Design review of the part built by this model. Coordinates are the model's own, in mm. Face numbers are marked on the shaded views. A direction names the side the tool comes from. Give positions to 0.01 mm unless a question says otherwise; leave off trailing zeros. Return JSON: item names as keys, results as strings.
```python
from build123d import *

# Parameters (mm, degrees)
F0_R      = 14.5
F1_DEPTH  = 10
F2_R      = 11.5
F3_DEPTH  = 9
F4_R      = 14.5
F4_R_2    = 11.5
F5_DEPTH  = 6
F6_R      = 25
F7_DEPTH  = 9
F8_R      = 1
F9_R      = 5.75
F10_DEPTH = 12.5
F11_R     = 3.75
F12_DEPTH = 8
F13_SIZE  = 0.5
F14_R     = 2.75
F15_DEPTH = 19


with BuildPart() as f1:
    # F0 (on Top) → F1 (new body)
    with BuildSketch(Plane.XY):
        Circle(F0_R)
    extrude(amount=F1_DEPTH)

    # F2 (on face) → F3 (join)
    with BuildSketch(Plane.XY.offset(10)):
        Circle(F2_R)
        with BuildLine():
            ThreePointArc((2, 7.7459666924), (5.6568542495, 5.6568542495), (7.7459666924, 2))
            Line((7.7459666924, 2), (8.3459666924, 2))
            ThreePointArc((8.3459666924, 2), (10.3459666924, 0), (8.3459666924, -2))
            Line((8.3459666924, -2), (7.7459666924, -2))
            ThreePointArc((7.7459666924, -2), (5.6568542495, -5.6568542495), (2, -7.7459666924))
            Line((2, -7.7459666924), (2, -8.3459666924))
            ThreePointArc((2, -8.3459666924), (0, -10.3459666924), (-2, -8.3459666924))
            Line((-2, -8.3459666924), (-2, -7.7459666924))
            ThreePointArc((-2, -7.7459666924), (-5.6568542495, -5.6568542495), (-7.7459666924, -2))
            Line((-7.7459666924, -2), (-8.3459666924, -2))
            ThreePointArc((-8.3459666924, -2), (-10.3459666924, 0), (-8.3459666924, 2))
            Line((-8.3459666924, 2), (-7.7459666924, 2))
            ThreePointArc((-7.7459666924, 2), (-5.6568542495, 5.6568542495), (-2, 7.7459666924))
            Line((-2, 7.7459666924), (-2, 8.3459666924))
            ThreePointArc((-2, 8.3459666924), (0, 10.3459666924), (2, 8.3459666924))
            Line((2, 8.3459666924), (2, 7.7459666924))
        make_face(mode=Mode.SUBTRACT)
    extrude(amount=F3_DEPTH)

    # F4 (on face) → F5 (join)
    with BuildSketch(Plane.XY.offset(10)):
        Circle(F4_R)
        Circle(F4_R_2, mode=Mode.SUBTRACT)
    extrude(amount=F5_DEPTH)

    # F6 (on face) → F7 (cut)
    with BuildSketch(Plane(origin=(0, 0, 0), x_dir=(1, 0, 0), z_dir=(0, 0, -1))):
        Circle(F6_R)
    extrude(amount=-F7_DEPTH, mode=Mode.SUBTRACT)

    # F8
    f8_edges = [f1.edges().sort_by_distance(p)[0] for p in [
        (-7.745967, 2, 14.5),
        (-2, 7.745967, 14.5),
        (2, 7.745967, 14.5),
        (7.745967, 2, 14.5),
        (-7.745967, -2, 14.5),
        (7.745967, -2, 14.5),
        (2, -7.745967, 14.5),
        (-2, -7.745967, 14.5),
    ]]
    fillet(f8_edges, radius=F8_R)

    # F9 (on face) → F10 (join)
    with BuildSketch(Plane.XY.offset(10)):
        Circle(F9_R)
    extrude(amount=F10_DEPTH)

    # F11 (on face) → F12 (join)
    with BuildSketch(Plane.XY.offset(22.5)):
        Circle(F11_R)
    extrude(amount=F12_DEPTH)

    # F13
    f13_edges = [f1.edges().sort_by_distance(p)[0] for p in [
        (-10.345967, 0, 19),
        (-7.889975, -2.194073, 19),
        (-7.889975, 2.194073, 19),
        (-5.656854, -5.656854, 19),
        (-5.656854, 5.656854, 19),
        (-2.194073, -7.889975, 19),
        (-2.194073, 7.889975, 19),
        (0, -10.345967, 19),
        (0, 10.345967, 19),
        (2.194073, -7.889975, 19),
        (2.194073, 7.889975, 19),
        (5.656854, -5.656854, 19),
        (5.656854, 5.656854, 19),
        (7.889975, -2.194073, 19),
        (7.889975, 2.194073, 19),
        (10.345967, 0, 19),
        (-11.5, 0, 19),
        (-14.5, 0, 16),
        (-3.75, 0, 30.5),
        (-5.75, 0, 22.5),
        (-14.5, 0, 9),
    ]]
    chamfer(f13_edges, length=F13_SIZE)

    # F14 (on face) → F15 (cut)
    with BuildSketch(Plane.XY.offset(30.5)):
        Circle(F14_R)
    extrude(amount=-F15_DEPTH, mode=Mode.SUBTRACT)


solid = f1.part
```
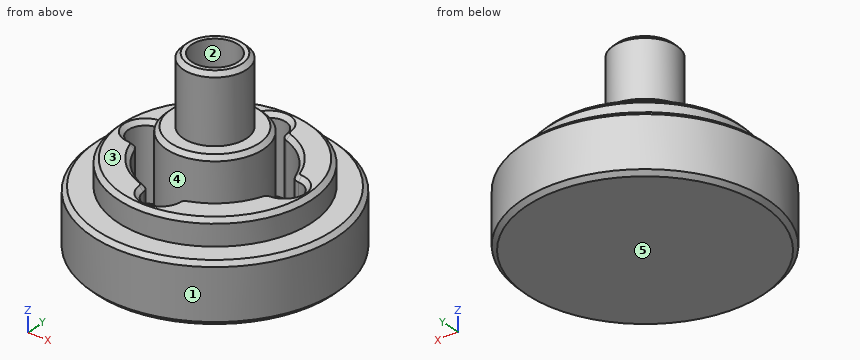
Item 1: Machinability: for the marked faces 4 and 5, which of the approach directions +Z, -Z, +X, -X, +Y, -Y give a long, thin tool a straight path to every point of the face, cutting with its end or side? Answer none if there is none.
Result set:
{"face 4": "+Z", "face 5": "-Z, +X, -X, +Y, -Y"}
Item 2: Mouldability with a two-part tool opening along Y and no side actions: class the marked faces 1, 2 and 3 as released by +Y, released by -Y, zero draft, split by the parting line, or undercut.
Result set:
{"face 1": "split by the parting line", "face 2": "undercut", "face 3": "zero draft"}
Item 3: Wall thickness on L1, parallel to Y at x = 0, z = 23; L2, parallel to Y at x = -3, z = 13.5; L3, parallel to Z at x = -10, y = -2: over which ranges is each line inside the solid? List them lowest first. Write a range as [from, to].
Result set:
{"L1": "y = [-3.75, -2.75], [2.75, 3.75]", "L2": "y = [-14.19, -7.42], [-4.91, 4.91], [7.42, 14.19]", "L3": "z = [9, 19]"}
Item 4: Add section A-A (z = 17). Give the number of separate pieces and of enclosed holes in the cut face, plus the area to 3 significant figures.
Result set:
{"separate pieces": "2", "enclosed holes": "2", "area": "262 mm^2"}
Item 5: For pin 1 (4 mm diameter, centred on x = 9, y = 0, fed in from +Z); pin 2 (1 mm diameter, centred on y = -7.5, z = 16, fed in from +X); pin 3 (4 mm diameter, centred on x = -1, z = 18.5, fed in from +Y); pin 4 (6 mm diameter, centred on x = 0, y = 0.5, fed in from +Z), all flat-tipped, find the tip position at first contact; note any pin that passes through.
Result set:
{"pin 1": "stops at z = 19", "pin 2": "stops at x = 12.48", "pin 3": "stops at y = 11.5", "pin 4": "stops at z = 30.5"}
